CAD build for the part. Positions are in the model's coordinates, mm. A direction names the side the tool comes from. Coordinates: 2 decimals unless noted, no trailing zeros. Loops run counter-clockwise (first coordinate to the right, second up) from the corner with the lowest first, then second, coordinate; pieces in that order, holes last. Notation, with made-up numbers: (6, 66) -> (58, 66) arc R23 ccw to (58, 104) -> close; hole circle Ø2 at (64, 29.5). An arc over 180 degrees is marked (long way). Write each question's results on one line, items separated by ' | '.
```python
from build123d import *

# Parameters (mm, degrees)
ESQUISSE1_W        = 50
ESQUISSE1_H        = 50
BOSS_EXTRU_1_DEPTH = 30
CONG_1_R           = 2


with BuildPart() as part:
    # Esquisse1 → Boss.-Extru.1 (new body)
    with BuildSketch(Plane(origin=(0, 0, 0), x_dir=(1, 0, 0), z_dir=(0, 1, 0))):
        with Locations((13.704515327, -15.337721188)):
            Rectangle(ESQUISSE1_W, ESQUISSE1_H)
        with BuildLine():
            Line((-3.295484673, 7.662278812), (30.704515327, 7.662278812))
            ThreePointArc((30.704515327, 7.662278812), (32.461874639, 3.419638124), (36.704515327, 1.662278812))
            Line((36.704515327, 1.662278812), (36.704515327, -32.337721188))
            ThreePointArc((36.704515327, -32.337721188), (32.461874639, -34.095080501), (30.704515327, -38.337721188))
            Line((30.704515327, -38.337721188), (-3.295484673, -38.337721188))
            ThreePointArc((-3.295484673, -38.337721188), (-5.052843986, -34.095080501), (-9.295484673, -32.337721188))
            Line((-9.295484673, -32.337721188), (-9.295484673, 1.662278812))
            ThreePointArc((-9.295484673, 1.662278812), (-5.052843986, 3.419638124), (-3.295484673, 7.662278812))
        make_face(mode=Mode.SUBTRACT)
    extrude(amount=BOSS_EXTRU_1_DEPTH)

    # Congé1
    cong_1_edges = [part.edges().sort_by_distance(p)[0] for p in [
        (-11.295484673, 15, -9.662278812),
        (38.704515327, 15, 40.337721188),
        (-11.295484673, 15, 40.337721188),
    ]]
    fillet(cong_1_edges, radius=CONG_1_R)


solid = part.part
```
Q1. Drop a flat-ended pin along its axis: pin 1 (12 mm diameter, centred on x = 1.5, z = 1.5, fed in from -Y). Give the stop position or say it passes through.
Results are:
pin 1: through
Q2. Which spindle directions (+Z, -Z, +X, -X, +Y, -Y) get a long thin tool onto all of the face, cutting with end or side? Do faces 4 (the cylindrical face through (-10.725, 15.21, -9.061)), 5 (the flat face through (36.705, 15, 15)). Say none if no direction does.
Results are:
face 4: -Z, -X, +Y, -Y | face 5: +Y, -Y
Q3. Pull direction Z, two halves, no side cores. Call faces 1 (the flat face through (13, 15, 40.338)), 2 (the cylindrical face through (-5.1, 14.79, -3.373)), 3 (the flat face through (14, 30, -9)): +Z half, -Z half, draft (parallel to the pull), parting line (faces both ways), or undercut.
Results are:
face 1: +Z half | face 2: undercut | face 3: draft
Q4. Cut at A-A on z = 28.5. Write the cut outline in (x, y).
Results are:
outline: (-11.3, 0) -> (-9.3, 0) -> (-9.3, 30) -> (-11.3, 30) -> close; (36.7, 0) -> (38.7, 0) -> (38.7, 30) -> (36.7, 30) -> close
Q5. Cut at B-B on x = 23. Write the cut outline in (y, z), and give its area (3 significant figures).
Results are:
outline: (0, -9.66) -> (30, -9.66) -> (30, -7.66) -> (0, -7.66) -> close; (0, 38.34) -> (30, 38.34) -> (30, 40.34) -> (0, 40.34) -> close | area: 120 mm^2
Q6. Wall check: L1, parallel to Z at x = 28.5, y = 23.25; L2, parallel to X at y = 20, z = 1; L3, parallel to Z at x = -9, y = 28.25 (3 decimals). Give the ranges that are in metal, low to high. Write a range as from..to.
Results are:
L1: -9.66..-7.66, 38.34..40.34 | L2: -11.3..-9.3, 36.7..38.7 | L3: -9.662..-1.67, 32.345..40.338
Q7. Cut at C-C on y = 2.25. Write the cut outline in (x, z), and give its area (3 significant figures).
Results are:
outline: (-11.3, -7.66) arc R2 ccw to (-9.3, -9.66) -> (38.7, -9.66) -> (38.7, 38.34) arc R2 ccw to (36.7, 40.34) -> (-9.3, 40.34) arc R2 ccw to (-11.3, 38.34) -> close; hole (-9.3, -1.66) arc R6 cw to (-3.3, -7.66) -> (30.7, -7.66) arc R6 cw to (36.7, -1.66) -> (36.7, 32.34) arc R6 cw to (30.7, 38.34) -> (-3.3, 38.34) arc R6 cw to (-9.3, 32.34) -> close | area: 495 mm^2
